Design review of the part built by this model. Coordinates are the model's own, in mm. Face numbers are marked on the shaded views. A direction names the side the tool comes from. Give positions to 0.01 mm unless a question says otherwise; leave off trailing zeros. Write each loop counter-clockwise with the first axis right and the second up, starting at its lowest first coordinate (ties: lowest second). Pieces come first, ordered by that corner, then holes. Notation, with made-up numbers: M 46,55 L 74,55 A7 cw 74,68 Z; hole C 44,0 d4. An arc over 180 degrees is marked long. Use one line per item in the form item = value. Start each with the question number.
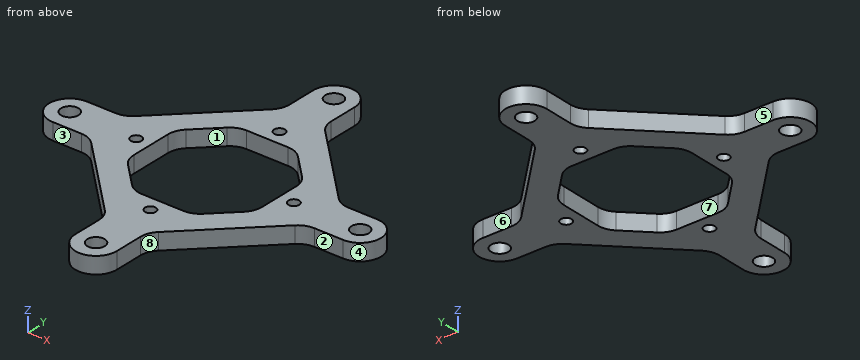
from build123d import *

# Parameters (mm, degrees)
SKETCH_1_R          = 2.1
SKETCH_1_W          = 10
SKETCH_1_H          = 10
EXTRUDE_1_DEPTH     = 4
CHAMFER_1_SIZE      = 21
SKETCH_2_R          = 1.3
CUT_EXTRUDE_1_DEPTH = 57.709787515
FILLET_3_R          = 5


with BuildPart() as part:
    # 草图1 → 凸台-拉伸1 (new body)
    # profile 1 of 5: a face of its own
    with BuildSketch(Plane.XY):
        with BuildLine():
            Line((5, 5), (5, 35))
            ThreePointArc((5, 35), (0, 40), (-5, 35))
            Line((-5, 35), (-5, 5))
            Line((-5, 5), (5, 5))
        make_face()
        with Locations((0, 35)):
            Circle(SKETCH_1_R, mode=Mode.SUBTRACT)
    # profile 2 of 5: a face of its own
    with BuildSketch(Plane.XY):
        with BuildLine():
            Line((5, -35), (5, -5))
            Line((5, -5), (-5, -5))
            Line((-5, -5), (-5, -35))
            ThreePointArc((-5, -35), (0, -40), (5, -35))
        make_face()
        with Locations((0, -35)):
            Circle(SKETCH_1_R, mode=Mode.SUBTRACT)
    # profile 3 of 5: a face of its own
    with BuildSketch(Plane.XY):
        Rectangle(SKETCH_1_W, SKETCH_1_H)
    # profile 4 of 5: a face of its own
    with BuildSketch(Plane.XY):
        with BuildLine():
            Line((35, 5), (5, 5))
            Line((5, 5), (5, -5))
            Line((5, -5), (35, -5))
            ThreePointArc((35, -5), (40, 0), (35, 5))
        make_face()
        with Locations((35, 0)):
            Circle(SKETCH_1_R, mode=Mode.SUBTRACT)
    # profile 5 of 5: a face of its own
    with BuildSketch(Plane.XY):
        with BuildLine():
            Line((-5, -5), (-5, 5))
            Line((-5, 5), (-35, 5))
            ThreePointArc((-35, 5), (-40, 0), (-35, -5))
            Line((-35, -5), (-5, -5))
        make_face()
        with Locations((-35, 0)):
            Circle(SKETCH_1_R, mode=Mode.SUBTRACT)
    extrude(amount=EXTRUDE_1_DEPTH)

    # 倒角1
    chamfer_1_edges = [part.edges().sort_by_distance(p)[0] for p in [
        (5, 5, 2),
        (5, -5, 2),
        (-5, -5, 2),
        (-5, 5, 2),
    ]]
    chamfer(chamfer_1_edges, length=CHAMFER_1_SIZE)

    # 草图2 → 切除-拉伸1 (cut, through all)
    with BuildSketch(Plane.XY.offset(4)):
        with Locations((0, 19)):
            Circle(SKETCH_2_R)
        with Locations((19, 0)):
            Circle(SKETCH_2_R)
        with Locations((0, -19)):
            Circle(SKETCH_2_R)
        with Locations((-19, 0)):
            Circle(SKETCH_2_R)
        Polygon((-7.071067812, 15.443650814), (-15.443650814, 7.071067812), (-15.443650814, -7.071067812), (-7.071067812, -15.443650814), (7.071067812, -15.443650814), (15.443650814, -7.071067812), (15.443650814, 7.071067812), (7.071067812, 15.443650814), align=None)
    extrude(amount=-CUT_EXTRUDE_1_DEPTH, mode=Mode.SUBTRACT)

    # 圆角3
    fillet_3_edges = [part.edges().sort_by_distance(p)[0] for p in [
        (15.443650814, -7.071067812, 2),
        (7.071067812, -15.443650814, 2),
        (-7.071067812, -15.443650814, 2),
        (-15.443650814, -7.071067812, 2),
        (-15.443650814, 7.071067812, 2),
        (-5, -26, 2),
        (-26, -5, 2),
        (26, -5, 2),
        (5, -26, 2),
        (5, 26, 2),
        (26, 5, 2),
        (-26, 5, 2),
        (-5, 26, 2),
        (-7.071067812, 15.443650814, 2),
        (7.071067812, 15.443650814, 2),
        (15.443650814, 7.071067812, 2),
    ]]
    fillet(fillet_3_edges, radius=FILLET_3_R)


solid = part.part
1. To check wall thickness, follow L1, parallel to Y at x = 0, z = 1.8; L2, parallel to Y at x = 35, z = 1.9; L3, parallel to X at y = 31.5, z = 1.05. State the ranges of each line that lie inside material, in increasing order.
2. We need section B-B (x = -13). State the section outline as (y, z) points, and give its area (3 significant figures).
3. For the marked faces 1, 2, 3, 4 and 5, list the 3-axis set-ups (+Z, -Z, +X, -X, +Y, -Y) from which the entire face can be reached by the end or side of a thin tool; tool diameter is ignored.
4. We need section A-A (y = 0). State the section outline as (x, z) points.
5. Clearance check with flat-ended pins moving along their axes: pin 1 Ø2 at (y, z) = (32.5, 2.5) entering from -X; pin 2 Ø2 at (x, z) = (-31, 2) entering from +Y; pin 3 Ø2 at (y, z) = (8, 1) entering from +X; pin 4 Ø2.5 at (x, y) = (0, 19) entering from -Z. State where each tip first meets the part, or that it passes through.
6. Draft analysis for pull direction Y (two halves, no side actions). For the marked faces 6, 7 and 8, state which applies: pulls with the +Y half, pulls with the -Y half, needs draft (parallel to the pull), parting line crosses it, or undercut.
7. We need section D-D (z = 2.4). Give the number of separate pieces and of enclosed holes in the cut face, and give its area (3 significant figures).
Answer block:
q1.L1 = -40 to -37.1, -32.9 to -20.3, -17.7 to -15.44, 15.44 to 17.7, 20.3 to 32.9, 37.1 to 40
q1.L2 = -5 to -2.1, 2.1 to 5
q1.L3 = -5 to 5
q2.outline = M -18,0 L -9.51,0 L -9.51,4 L -18,4 Z; M 9.51,0 L 18,0 L 18,4 L 9.51,4 Z
q2.area = 67.9 mm^2
q3.face_1 = +Z, -Z
q3.face_2 = +Z, -Z, +X, -Y
q3.face_3 = +Z, -Z, -X, -Y
q3.face_4 = +Z, -Z, +X
q3.face_5 = +Z, -Z, -X, +Y
q4.outline = M -40,0 L -37.1,0 L -37.1,4 L -40,4 Z; M -32.9,0 L -20.3,0 L -20.3,4 L -32.9,4 Z; M -17.7,0 L -15.44,0 L -15.44,4 L -17.7,4 Z; M 15.44,0 L 17.7,0 L 17.7,4 L 15.44,4 Z; M 20.3,0 L 32.9,0 L 32.9,4 L 20.3,4 Z; M 37.1,0 L 40,0 L 40,4 L 37.1,4 Z
q5.pin_1 = -5
q5.pin_2 = 5
q5.pin_3 = 24
q5.pin_4 = through
q6.face_6 = pulls with the +Y half
q6.face_7 = undercut
q6.face_8 = pulls with the -Y half
q7.separate_pieces = 1
q7.enclosed_holes = 9
q7.area = 1,460 mm^2
